```python
from build123d import *

# Parameters (mm, degrees)
SKETCH1_R           = 18.5
BOSS_EXTRUDE1_DEPTH = 70
SKETCH2_R           = 1.9
CUT_EXTRUDE1_DEPTH  = 3
SKETCH2_3_R         = 6
BOSS_EXTRUDE2_DEPTH = 6
SKETCH3_R           = 3
BOSS_EXTRUDE3_DEPTH = 20


with BuildPart() as part:
    # Sketch1 → Boss-Extrude1 (new body)
    with BuildSketch(Plane(origin=(0, 0, 0), x_dir=(0, 1, 0), z_dir=(0, 0, 1))):
        with Locations(Location((0, 0, 0), (0, 0, 270))):
            Circle(SKETCH1_R)
    extrude(amount=BOSS_EXTRUDE1_DEPTH)

    # Sketch2 → Cut-Extrude1 (cut)
    with BuildSketch(Plane(origin=(0, 0, 70), x_dir=(-1, 0, 0), z_dir=(0, 0, 1))):
        with Locations(Location((-15.5, 0, 0), (0, 0, 180))):
            Circle(SKETCH2_R)
        with Locations(Location((-7.75, 13.423393759, 0), (0, 0, 180))):
            Circle(SKETCH2_R)
        with Locations(Location((7.75, 13.423393759, 0), (0, 0, 180))):
            Circle(SKETCH2_R)
        with Locations(Location((15.5, 0, 0), (0, 0, 180))):
            Circle(SKETCH2_R)
        with Locations(Location((7.75, -13.423393759, 0), (0, 0, 180))):
            Circle(SKETCH2_R)
        with Locations(Location((-7.75, -13.423393759, 0), (0, 0, 180))):
            Circle(SKETCH2_R)
    extrude(amount=-CUT_EXTRUDE1_DEPTH, mode=Mode.SUBTRACT)

    # Sketch2_3 → Boss-Extrude2 (add)
    with BuildSketch(Plane(origin=(0, 0, 70), x_dir=(-1, 0, 0), z_dir=(0, 0, 1))):
        with Locations(Location((0, -7, 0), (0, 0, 180))):
            Circle(SKETCH2_3_R)
    extrude(amount=BOSS_EXTRUDE2_DEPTH)

    # Sketch3 → Boss-Extrude3 (add)
    with BuildSketch(Plane.XY.offset(76)):
        with Locations((0, 7)):
            Circle(SKETCH3_R)
    extrude(amount=BOSS_EXTRUDE3_DEPTH)


solid = part.part
```
Geometry check sheet. Reference: the model listing, model coordinates, mm. A direction names the side the tool comes from. Coordinates: 2 decimals unless noted, no trailing zeros. Order: outer loops, then holes, each group sorted by start corner. A loop starts at its lowest first (then second) coordinate and runs counter-clockwise, first axis right, second up. Notation, with made-up numbers: (77, -37.5) - (119, -37.5) arc R23 cw to (119, -8.5) - close; hole circle Ø8 at (58, 87.25). An arc over 180 degrees is marked (long way). Answer in a Markdown table with one row per item. Add a question column.
1. Draft check along X on faces 3 (the face through (13.6, 0.08, 68.52)), 4 (the face through (-0.78, 12.95, 72.96)), 5 (the face through (0, 0, 70)). Enter one of: +X half, -X half, draft (parallel to the pull), parting line (faces both ways), or undercut.
2. Gauge pin test, flat ends, axial feed: pin 1 Ø2 at (x, z) = (4.5, 46) entering from +Y; pin 2 Ø2.5 at (x, y) = (7.75, -13.42) entering from +Z; pin 3 Ø12 at (y, z) = (-12.5, 51) entering from +X. Record the tip position at first contact, or that the pin passes through.
3. Section check B-B (z = 47). Enter the section's corners in (x, y), plus the area to 3 significant figures.
4. Section check D-D (x = 8). Enter the section's corners in (y, z), plus the area to 3 significant figures.
5. Material ranges on L1, parallel to Y at x = -7.75, z = 68.4; L2, parallel to Z at x = 8, y = -6.5; L3, parallel to Y at x = -7, z = 69, recorded low to high. Write a range as [from, to].
6. Section check C-C (y = -3.5). Enter the section's corners in (x, z), plus the area to 3 significant figures.
7. Section check A-A (x = 0). Enter the section's corners in (y, z), plus the area to 3 significant figures.
8. Access from +Z, -Z, +X, -X, +Y, -Y to the whole of each face (thin tool, end or side, straight path). Record for faces 1 (the face through (15, 0, 67)), 2 (the face through (0, 0, 0)).
Data:
| question | item | result |
|---|---|---|
| 1 | face 3 | undercut |
| 1 | face 4 | parting line |
| 1 | face 5 | draft |
| 2 | pin 1 | stops at y = 18.17 |
| 2 | pin 2 | stops at z = 67 |
| 2 | pin 3 | stops at x = 17.32 |
| 3 | outline | circle Ø37 at (0, 0) |
| 3 | area | 1,080 mm² |
| 4 | outline | (-16.68, 0) - (16.68, 0) - (16.68, 70) - (15.31, 70) - (15.31, 67) - (11.54, 67) - (11.54, 70) - (-11.54, 70) - (-11.54, 67) - (-15.31, 67) - (-15.31, 70) - (-16.68, 70) - close |
| 4 | area | 2,310 mm² |
| 5 | L1 | y = [-16.8, -15.32], [-11.52, 11.52], [15.32, 16.8] |
| 5 | L2 | z = [0, 70] |
| 5 | L3 | y = [-17.12, -15.17], [-11.68, 11.68], [15.17, 17.12] |
| 6 | outline | (-18.17, 0) - (18.17, 0) - (18.17, 70) - (-18.17, 70) - close |
| 6 | area | 2,540 mm² |
| 7 | outline | (-18.5, 0) - (18.5, 0) - (18.5, 70) - (13, 70) - (13, 76) - (10, 76) - (10, 96) - (4, 96) - (4, 76) - (1, 76) - (1, 70) - (-18.5, 70) - close |
| 7 | area | 2,780 mm² |
| 8 | face 1 | +Z |
| 8 | face 2 | -Z, +X, -X, +Y, -Y |
